```python
from build123d import *

# Parameters (mm, degrees)
F0_W      = 790
F0_H      = 75
F1_DEPTH  = 170
F2_W      = 40
F2_H      = 55
F3_DEPTH  = 150
F5_DEPTH  = 25
F4_W      = 40
F4_H      = 5
F6_DEPTH  = 23
F7_W      = 40
F7_H      = 5
F8_DEPTH  = 23
F10_DEPTH = 25
F12_DEPTH = 27
F13_W     = 40
F13_H     = 5
F14_DEPTH = 20
F15_W     = 40
F15_H     = 30
F16_DEPTH = 5


with BuildPart() as f1:
    # F0 (on Front) → F1 (new body)
    with BuildSketch(Plane.XZ):
        with Locations((-9.780855, -37.5)):
            Rectangle(F0_W, F0_H)
    extrude(amount=F1_DEPTH)

    # F2 (on face) → F3 (cut)
    with BuildSketch(Plane.XZ.offset(170)):
        with Locations((-361.780855, -47.5)):
            Rectangle(F2_W, F2_H)
        with Locations((-297.780855, -47.5)):
            Rectangle(F2_W, F2_H)
        with Locations((-233.780855, -47.5)):
            Rectangle(F2_W, F2_H)
        with Locations((-169.780855, -47.5)):
            Rectangle(F2_W, F2_H)
        with Locations((-105.780855, -47.5)):
            Rectangle(F2_W, F2_H)
        with Locations((-41.780855, -47.5)):
            Rectangle(F2_W, F2_H)
        with Locations((22.219145, -47.5)):
            Rectangle(F2_W, F2_H)
        with Locations((86.219145, -47.5)):
            Rectangle(F2_W, F2_H)
        with Locations((150.219145, -47.5)):
            Rectangle(F2_W, F2_H)
        with Locations((214.219145, -47.5)):
            Rectangle(F2_W, F2_H)
        with Locations((278.219145, -47.5)):
            Rectangle(F2_W, F2_H)
        with Locations((342.219145, -47.5)):
            Rectangle(F2_W, F2_H)
    extrude(amount=-F3_DEPTH, mode=Mode.SUBTRACT)

    # F4 (on face) → F5 (cut)
    with BuildSketch(Plane(origin=(-404.780855, 0, 0), x_dir=(0, -1, 0), z_dir=(-1, 0, 0))):
        Polygon((106.5, 0), (85, 0), (63.5, 0), (63.5, -7), (106.5, -7), align=None)
    extrude(amount=-F5_DEPTH, mode=Mode.SUBTRACT)

    # F4 (on face) → F6 (join)
    with BuildSketch(Plane(origin=(-404.780855, 0, 0), x_dir=(0, -1, 0), z_dir=(-1, 0, 0))):
        with Locations((85, -77.5)):
            Rectangle(F4_W, F4_H)
    extrude(amount=-F6_DEPTH)

    # F7 (on face) → F8 (join)
    with BuildSketch(Plane.YZ.offset(385.219145)):
        with Locations((-85, -77.5)):
            Rectangle(F7_W, F7_H)
    extrude(amount=-F8_DEPTH)

    # F9 (on face) → F10 (cut)
    with BuildSketch(Plane.YZ.offset(385.219145)):
        Polygon((-63.5, 0), (-85, 0), (-106.5, 0), (-106.5, -7), (-63.5, -7), align=None)
    extrude(amount=-F10_DEPTH, mode=Mode.SUBTRACT)

    # F11 (on face) → F12 (cut)
    with BuildSketch(Plane(origin=(0, 0, 0), x_dir=(-1, 0, 0), z_dir=(0, 1, 0))):
        Polygon((31.280855, 0), (9.780855, 0), (-11.719145, 0), (-11.719145, -7), (31.280855, -7), align=None)
    extrude(amount=-F12_DEPTH, mode=Mode.SUBTRACT)

    # F13 (on face) → F14 (join)
    with BuildSketch(Plane(origin=(0, 0, 0), x_dir=(-1, 0, 0), z_dir=(0, 1, 0))):
        with Locations((9.780855, -77.5)):
            Rectangle(F13_W, F13_H)
    extrude(amount=-F14_DEPTH)

    # F15 (on face) → F16 (cut)
    with BuildSketch(Plane(origin=(0, 0, -20), x_dir=(1, 0, 0), z_dir=(0, 0, -1))):
        with Locations((-361.780855, 35)):
            Rectangle(F15_W, F15_H)
        with Locations((-297.780855, 35)):
            Rectangle(F15_W, F15_H)
        with Locations((-233.780855, 35)):
            Rectangle(F15_W, F15_H)
        with Locations((-169.780855, 35)):
            Rectangle(F15_W, F15_H)
        with Locations((-105.780855, 35)):
            Rectangle(F15_W, F15_H)
        with Locations((-41.780855, 35)):
            Rectangle(F15_W, F15_H)
        with Locations((22.219145, 35)):
            Rectangle(F15_W, F15_H)
        with Locations((86.219145, 35)):
            Rectangle(F15_W, F15_H)
        with Locations((150.219145, 35)):
            Rectangle(F15_W, F15_H)
        with Locations((214.219145, 35)):
            Rectangle(F15_W, F15_H)
        with Locations((278.219145, 35)):
            Rectangle(F15_W, F15_H)
        with Locations((342.219145, 35)):
            Rectangle(F15_W, F15_H)
    extrude(amount=-F16_DEPTH, mode=Mode.SUBTRACT)


solid = f1.part
```
Check sheet for the modelled part. Datum: model origin and axes. Units: mm. A direction names the side the tool comes from. Coordinates: 2 decimals unless noted, no trailing zeros. Loops run counter-clockwise (first coordinate to the right, second up) from the corner with the lowest first, then second, coordinate; pieces in that order, holes last.
1) Sectioned sample at B-B (x = -233). Record the boundary of the cut face in (y, z), and give its area (3 significant figures).
2) Sectioned sample at A-A (y = -11.5). Record the boundary of the cut face in (x, z), and give its area (3 significant figures).
3) Gauge pin test, flat ends, axial feed: pin 1 (20 mm diameter, centred on x = 19, y = -113, fed in from -Z); pin 2 (5.5 mm diameter, centred on x = 376.5, z = -3.5, fed in from +Y); pin 3 (5 mm diameter, centred on x = 4.5, y = -36, fed in from -Z); pin 4 (4 mm diameter, centred on x = 376, z = -77.5, fed in from -Y). Record the tip position at first contact, or that the pin passes through.
4) Sectioned sample at C-C (x = 58). Record the boundary of the cut face in (y, z), and give its area (4 significant figures).
5) Release check for a two-part mould opening along X. For faces 4 (the face through (-277.781, -96, -45)), 5 (the face through (374, -137, -75)) record: released by +X, released by -X, zero draft, split by the parting line, or undercut.
6) Access from +Z, -Z, +X, -X, +Y, -Y to the whole of each face (thin tool, end or side, straight path). Record for faces 1 (the face through (-42, -35, -15)), 2 (the face through (373, -85, -7)), 3 (the face through (-234, -111, -20)).
7) Material ranges on probe 1 along Z at (x, y) = (253.5, -34.5); probe 2 along Y at (x, z) = (324, -27.5), recorded low to high.
Check sheet entries:
1. outline: (-170, -20) - (-50, -20) - (-50, -15) - (-20, -15) - (-20, -75) - (0, -75) - (0, 0) - (-170, 0) - close
1. area: 4,350 mm2
2. outline: (-404.78, -75) - (-29.78, -75) - (-29.78, -80) - (10.22, -80) - (10.22, -75) - (385.22, -75) - (385.22, 0) - (11.72, 0) - (11.72, -7) - (-31.28, -7) - (-31.28, 0) - (-404.78, 0) - close
2. area: 59,100 mm2
3. pin 1: stops at z = -20
3. pin 2: stops at y = 0
3. pin 3: stops at z = -75
3. pin 4: stops at y = -105
4. outline: (-170, -75) - (0, -75) - (0, 0) - (-170, 0) - close
4. area: 12,750 mm2
5. face 4: undercut
5. face 5: zero draft
6. face 1: -Z
6. face 2: +Z, +X
6. face 3: -Z, -Y
7. probe 1: z = -75 to 0
7. probe 2: y = -20 to 0
